Can you work these out from the model? Positions are in its coordinate system, mm. Face numbers are marked on the shaded views. A direction names the side the tool comes from. Give positions to 0.01 mm unless a question says otherwise; leave off trailing zeros. Loops run counter-clockwise (first coordinate to the right, second up) from the corner with the lowest first, then second, coordinate; pieces in that order, holes last. Notation, with made-up numbers: (77, -21.5) - (119, -21.5) arc R33 ccw to (119, 6.5) - close; hole circle Ø8 at (-19, -26.75). An arc over 180 degrees is marked (long way). Answer in a Markdown table with one row per item.
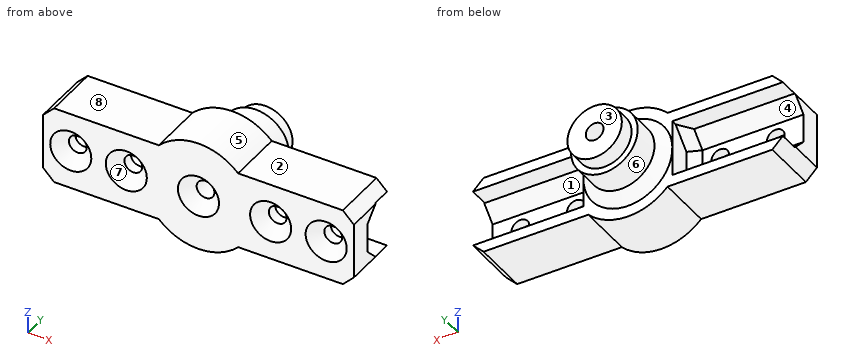
from build123d import *

# Parameters (mm, degrees)
BOSS_EXTRU_1_DEPTH           = 10
ENL_V_MAT_EXTRU_1_DEPTH      = 20
CHANFREIN1_SIZE              = 2.5
CHANFREIN2_SIZE              = 1.8
CHANFREIN1_OF_SYM_TRIE1_SIZE = 2.5
CHANFREIN2_OF_SYM_TRIE1_SIZE = 1.8
ESQUISSE5_R                  = 1.6000000000000016
ESQUISSE5_R_2                = 1.6000000000000019
ENL_V_MAT_EXTRU_4_DEPTH      = 7
CHANFREIN4_SIZE              = 2.1
CHANFREIN5_SIZE              = 2
ESQUISSE6_R                  = 6
BOSS_EXTRU_2_DEPTH           = 7
ESQUISSE7_R                  = 4.9
BOSS_EXTRU_3_DEPTH           = 2.9
ESQUISSE8_R                  = 1.6
ENL_V_MAT_EXTRU_5_DEPTH      = 36.777227393972275
CHANFREIN6_SIZE              = 2.1
CHANFREIN7_SIZE              = 2


with BuildPart() as part:
    # Esquisse1 → Boss.-Extru.1 (new body)
    with BuildSketch(Plane(origin=(0, 0, 0), x_dir=(1, 0, 0), z_dir=(0, 1, 0))):
        with BuildLine():
            Line((7.1414284285428495, 7), (27.999999999999996, 7))
            Line((27.999999999999996, 7), (27.999999999999996, -7))
            Line((27.999999999999996, -7), (7.1414284285428495, -7))
            ThreePointArc((7.1414284285428495, -7), (6.1e-16, -10), (-7.1414284285428495, -7))
            Line((-7.1414284285428495, -7), (-28.000000000000004, -7))
            Line((-28.000000000000004, -7), (-28.000000000000004, 7))
            Line((-28.000000000000004, 7), (-7.1414284285428495, 7))
            ThreePointArc((-7.1414284285428495, 7), (6.1e-16, 10), (7.1414284285428495, 7))
        make_face()
    extrude(amount=BOSS_EXTRU_1_DEPTH)

    # Esquisse2 → Enlèv. mat.-Extru.1 (cut)
    with BuildSketch(Plane.ZY.offset(28.000000000000004)):
        Polygon((-5.1000000000000005, 10), (5.099999999999999, 10), (5.099999999999999, 3.999999999999999), (-5.1000000000000005, 4), align=None)
    enl_v_mat_extru_1 = extrude(amount=-ENL_V_MAT_EXTRU_1_DEPTH, mode=Mode.SUBTRACT)

    # Chanfrein1
    chanfrein1_edges = [part.edges().sort_by_distance(p)[0] for p in [
        (-18.000000000000004, 4, -5.1000000000000005),
        (-18.000000000000004, 3.999999999999999, 5.099999999999999),
    ]]
    chamfer(chanfrein1_edges, length=CHANFREIN1_SIZE)

    # Chanfrein2
    chanfrein2_edges = [part.edges().sort_by_distance(p)[0] for p in [
        (-8.000000000000004, 3.9999999999999996, -8.9e-16),
        (-8.000000000000005, 5.250000000000001, -3.8500000000000005),
        (-8.000000000000004, 5.25, 3.849999999999998),
    ]]
    chamfer(chanfrein2_edges, length=CHANFREIN2_SIZE)

    # Symétrie1: Enlèv. mat.-Extru.1 across plane
    add(enl_v_mat_extru_1.mirror(Plane(origin=(0, 0, 0), x_dir=(0, 0, 1), z_dir=(1, 0, 0))), mode=Mode.SUBTRACT)

    # Chanfrein1 of Symétrie1
    chanfrein1_of_sym_trie1_edges = [part.edges().sort_by_distance(p)[0] for p in [
        (18.000000000000004, 4, -5.1000000000000005),
        (18.000000000000004, 3.999999999999999, 5.099999999999999),
    ]]
    chamfer(chanfrein1_of_sym_trie1_edges, length=CHANFREIN1_OF_SYM_TRIE1_SIZE)

    # Chanfrein2 of Symétrie1
    chanfrein2_of_sym_trie1_edges = [part.edges().sort_by_distance(p)[0] for p in [
        (8.000000000000004, 3.9999999999999996, -8.9e-16),
        (8.000000000000005, 5.250000000000001, -3.8500000000000005),
        (8.000000000000004, 5.25, 3.849999999999998),
    ]]
    chamfer(chanfrein2_of_sym_trie1_edges, length=CHANFREIN2_OF_SYM_TRIE1_SIZE)

    # Esquisse5 → Enlèv. mat.-Extru.4 (cut)
    with BuildSketch(Plane.XZ):
        with Locations(Location((-23.000000000000004, 0, 0), (0, 0, 270))):
            Circle(ESQUISSE5_R)
        with Locations(Location((-13.000000000000004, 0, 0), (0, 0, 270))):
            Circle(ESQUISSE5_R_2)
        with Locations(Location((12.999999999999996, 0, 0), (0, 0, 270))):
            Circle(ESQUISSE5_R_2)
        with Locations(Location((22.999999999999993, 0, 0), (0, 0, 270))):
            Circle(ESQUISSE5_R)
    extrude(amount=-ENL_V_MAT_EXTRU_4_DEPTH, mode=Mode.SUBTRACT)

    # Chanfrein4
    chanfrein4_edges = [part.edges().sort_by_distance(p)[0] for p in [
        (-23.000000000000004, 0, 1.6000000000000016),
        (-13.000000000000004, 0, 1.6000000000000019),
        (12.999999999999996, 0, 1.6000000000000019),
        (22.999999999999993, 0, 1.6000000000000016),
    ]]
    chamfer(chanfrein4_edges, length=CHANFREIN4_SIZE)

    # Chanfrein5
    chanfrein5_edges = [part.edges().sort_by_distance(p)[0] for p in [
        (27.999999999999996, 5, -7),
        (27.999999999999996, 5, 7),
        (-28.000000000000004, 5, -7),
        (-28.000000000000004, 5, 7),
    ]]
    chamfer(chanfrein5_edges, length=CHANFREIN5_SIZE)

    # Esquisse6 → Boss.-Extru.2 (add)
    with BuildSketch(Plane(origin=(0, 10, 0), x_dir=(1, 0, 0), z_dir=(0, 1, 0))):
        with Locations(Location((0, 0, 0), (0, 0, 270))):
            Circle(ESQUISSE6_R)
    extrude(amount=BOSS_EXTRU_2_DEPTH)

    # Esquisse7 → Boss.-Extru.3 (add)
    with BuildSketch(Plane(origin=(0, 17, 0), x_dir=(1, 0, 0), z_dir=(0, 1, 0))):
        with Locations(Location((0, 0, 0), (0, 0, 270))):
            Circle(ESQUISSE7_R)
    extrude(amount=BOSS_EXTRU_3_DEPTH)

    # Esquisse8 → Enlèv. mat.-Extru.5 (cut, through all)
    with BuildSketch(Plane(origin=(0, 19.900000000000002, 0), x_dir=(1, 0, 0), z_dir=(0, 1, 0))):
        with Locations(Location((0, 0, 0), (0, 0, 270))):
            Circle(ESQUISSE8_R)
    extrude(amount=-ENL_V_MAT_EXTRU_5_DEPTH, mode=Mode.SUBTRACT)

    # Chanfrein6
    chanfrein6_edges = [part.edges().sort_by_distance(p)[0] for p in [
        (4.9e-16, 0, -1.6),
    ]]
    chamfer(chanfrein6_edges, length=CHANFREIN6_SIZE)

    # Chanfrein7
    chanfrein7_edges = [part.edges().sort_by_distance(p)[0] for p in [
        (1.84e-15, 10, -6),
    ]]
    chamfer(chanfrein7_edges, length=CHANFREIN7_SIZE)


solid = part.part
Q1. For pin 1 (10 mm diameter, centred on x = -18.5, z = 3.5, fed in from +Y); pin 2 (1.6 mm diameter, centred on x = -21, z = 0.5, fed in from +Y); pin 3 (4.5 mm diameter, centred on y = 8, z = -1, fed in from -X), each with a flat end and sliding along its axis, tell me the tip position at first contact or that it passes through.
Checked values:
| item | result |
|---|---|
| pin 1 | stops at y = 10 |
| pin 2 | stops at y = 4 |
| pin 3 | stops at x = -8.09 |
Q2. If we mould it in two halves opening along Z, with no side actions, what happens to the marked faces 6, 7 and 8? For each: released by +Z, released by -Z, zero draft, split by the parting line, or undercut.
Checked values:
| item | result |
|---|---|
| face 6 | split by the parting line |
| face 7 | undercut |
| face 8 | released by +Z |
Q3. Imagine slicing it at B-B, the plane x = 0. Write out the boundary of the cut face in (y, z), and give its area (3 significant figures).
Checked values:
| item | result |
|---|---|
| outline | (0, -10) - (10, -10) - (10, -8) - (12, -6) - (17, -6) - (17, -4.9) - (19.9, -4.9) - (19.9, -1.6) - (2.1, -1.6) - (0, -3.7) - close; (0, 3.7) - (2.1, 1.6) - (19.9, 1.6) - (19.9, 4.9) - (17, 4.9) - (17, 6) - (12, 6) - (10, 8) - (10, 10) - (0, 10) - close |
| area | 248 mm² |
Q4. If I drill on line 1 (X direction, y = 2.85, z = 0); line 2 (X direction, y = 7.25, z = 0); line 3 (Z direction, x = 20.5, y = 7.5), over which ranges is the centre line in solid material (lowest first)? Write a range as [from, to].
Checked values:
| item | result |
|---|---|
| line 1 | x = [-28, -24.6], [-21.4, -14.6], [-11.4, -1.6], [1.6, 11.4], [14.6, 21.4], [24.6, 28] |
| line 2 | x = [-8, -1.6], [1.6, 8] |
| line 3 | z = [-7, -5.1], [5.1, 7] |
Q5. Imagine slicing it at C-C, the plane y = 8.25. Write out the boundary of the cut face in (x, z), and give its area (3 significant figures).
Checked values:
| item | result |
|---|---|
| outline | (-27.9, -5.1) - (-26, -7) - (-7.14, -7) arc R10 ccw to (7.14, -7) - (26, -7) - (27.9, -5.1) - (8.56, -5.1) - (8, -4.3) - (8, 4.3) - (8.56, 5.1) - (27.9, 5.1) - (26, 7) - (7.14, 7) arc R10 ccw to (-7.14, 7) - (-26, 7) - (-27.9, 5.1) - (-8.56, 5.1) - (-8, 4.3) - (-8, -4.3) - (-8.56, -5.1) - close; hole circle Ø3.2 at (0, 0) |
| area | 420 mm² |
Q6. Imagine slicing it at A-A, the plane x = -23. Write out the boundary of the cut face in (y, z).
Checked values:
| item | result |
|---|---|
| outline | (0, -7) - (10, -7) - (10, -5.1) - (6.5, -5.1) - (4, -2.6) - (4, -1.6) - (2.1, -1.6) - (0, -3.7) - close; (0, 3.7) - (2.1, 1.6) - (4, 1.6) - (4, 2.6) - (6.5, 5.1) - (10, 5.1) - (10, 7) - (0, 7) - close |
Q7. Imagine slicing it at D-D, the plane y = 13.5. Write out the boundary of the cut face in (x, z).
Checked values:
| item | result |
|---|---|
| outline | circle Ø12 at (0, 0); hole circle Ø3.2 at (0, 0) |
Q8. On a 3-axis mill with a long thin cutter (end or side, diameter ignored), from which of +Z, -Z, +X, -X, +Y, -Y can I reach the whole of each face in a straight line? I mean the marked faces 1, 2, 3, 4 and 5. Say none if no direction works.
Checked values:
| item | result |
|---|---|
| face 1 | +X, +Y |
| face 2 | +Z, +X, +Y, -Y |
| face 3 | +Z, -Z, +X, -X, +Y |
| face 4 | -X, +Y |
| face 5 | +Z, +Y, -Y |
